from build123d import *

# Parameters (mm, degrees)
SKETCH2_R           = 13.5
BOSS_EXTRUDE1_DEPTH = 8
SKETCH5_R           = 2.3
CUT_EXTRUDE4_DEPTH  = 10
SKETCH8_W           = 10
SKETCH8_H           = 1
CUT_EXTRUDE5_DEPTH  = 1
SKETCH11_R          = 3.5
CUT_EXTRUDE6_DEPTH  = 4.32
SKETCH12_R          = 1.27
CUT_EXTRUDE7_DEPTH  = 32.5


with BuildPart() as part:
    # Sketch2 → Boss-Extrude1 (new body)
    with BuildSketch(Plane.XY):
        Circle(SKETCH2_R)
    extrude(amount=BOSS_EXTRUDE1_DEPTH)

    # Sketch5 → Cut-Extrude4 (cut)
    with BuildSketch(Plane.XY.offset(8)):
        with Locations((0, 8)):
            Circle(SKETCH5_R)
    cut_extrude4 = extrude(amount=-CUT_EXTRUDE4_DEPTH, mode=Mode.SUBTRACT)

    # Mirror1: Cut-Extrude4 across plane
    add(cut_extrude4.mirror(Plane.ZX), mode=Mode.SUBTRACT)

    # Sketch8 → Cut-Extrude5 (cut)
    with BuildSketch(Plane(origin=(0, 0, 0), x_dir=(-1, 0, 0), z_dir=(0, 0, -1))):
        with Locations((-13.5, 0)):
            Rectangle(SKETCH8_W, SKETCH8_H)
    cut_extrude5 = extrude(amount=-CUT_EXTRUDE5_DEPTH, mode=Mode.SUBTRACT)

    # Mirror2: Cut-Extrude5 across plane
    add(cut_extrude5.mirror(Plane(origin=(0, 0, 0), x_dir=(0, 0, 1), z_dir=(1, 0, 0))), mode=Mode.SUBTRACT)

    # Sketch11 → Cut-Extrude6 (cut)
    with BuildSketch(Plane.XY.offset(8)):
        with Locations((0, 8)):
            Circle(SKETCH11_R)
    cut_extrude6 = extrude(amount=-CUT_EXTRUDE6_DEPTH, mode=Mode.SUBTRACT)

    # Mirror3: Cut-Extrude6 across plane
    add(cut_extrude6.mirror(Plane.ZX), mode=Mode.SUBTRACT)

    # Sketch12 → Cut-Extrude7 (cut)
    with BuildSketch(Plane.XY.offset(8)):
        with Locations((4.89, 0)):
            Circle(SKETCH12_R)
        with Locations((-4.89, 0)):
            Circle(SKETCH12_R)
    extrude(amount=-CUT_EXTRUDE7_DEPTH, mode=Mode.SUBTRACT)


solid = part.part
Design review of the part built by this model. Coordinates are the model's own, in mm. A direction names the side the tool comes from. Give positions to 0.01 mm unless a question says otherwise; leave off trailing zeros. Loops run counter-clockwise (first coordinate to the right, second up) from the corner with the lowest first, then second, coordinate; pieces in that order, holes last. Notation, with made-up numbers: M 20,73.5 L 36,73.5 A24 ccw 36,92.5 Z; hole C -32,36.5 d8. An arc over 180 degrees is marked long. Answer as a JSON object with one key per item and string values.
Item 1: Mouldability with a two-part tool opening along Y and no side actions: class faces 5 (the face through (0, 0, 0)), 6 (the face through (11, 0, 1)), 7 (the face through (-2.93, -13.18, 3.94)) as pulls with the +Y half, pulls with the -Y half, needs draft (parallel to the pull), parting line crosses it, or undercut.
Output values:
{"face 5": "needs draft", "face 6": "undercut", "face 7": "parting line crosses it"}
Item 2: Wall thickness on line 1 along Y through (x, z) = (0, 2.5); line 2 along Y through (x, z) = (0, 5.35); line 3 along X through (y, z) = (5.25, 5.75): over which ranges is each line inside the solid? List them lowest first.
Output values:
{"line 1": "y = -13.5 to -10.3, -5.7 to 5.7, 10.3 to 13.5", "line 2": "y = -13.5 to -11.5, -4.5 to 4.5, 11.5 to 13.5", "line 3": "x = -12.44 to -2.17, 2.17 to 12.44"}
Item 3: Machinability: for faces 1 (the face through (8.5, 0, 0.5)), 2 (the face through (-11, 0, 1)), 3 (the face through (-0.759, 4.583, 5.87)), 4 (the face through (-3.68, 0.38, 4.06)), which of the approach directions +Z, -Z, +X, -X, +Y, -Y give a long, thin tool a straight path to every point of the face, cutting with its end or side? Answer none if there is none.
Output values:
{"face 1": "-Z, +X", "face 2": "-Z, -X", "face 3": "+Z", "face 4": "+Z, -Z"}
Item 4: We need section D-D (x = -5.75). State the section outline as (y, z) points.
Output values:
{"outline": "M -12.21,0 L -0.93,0 L -0.93,8 L -12.21,8 Z; M 0.93,0 L 12.21,0 L 12.21,8 L 0.93,8 Z"}
Item 5: We need section A-A (x = 0). State the section outline as (y, z) points, and give its area (3 significant figures).
Output values:
{"outline": "M -13.5,0 L -10.3,0 L -10.3,3.68 L -11.5,3.68 L -11.5,8 L -13.5,8 Z; M -5.7,0 L 5.7,0 L 5.7,3.68 L 4.5,3.68 L 4.5,8 L -4.5,8 L -4.5,3.68 L -5.7,3.68 Z; M 10.3,0 L 13.5,0 L 13.5,8 L 11.5,8 L 11.5,3.68 L 10.3,3.68 Z", "area": "122 mm2"}
Item 6: We need section B-B (y = 0). State the section outline as (x, z) points.
Output values:
{"outline": "M -13.5,1 L -8.5,1 L -8.5,0 L -6.16,0 L -6.16,8 L -13.5,8 Z; M -3.62,0 L 3.62,0 L 3.62,8 L -3.62,8 Z; M 6.16,0 L 8.5,0 L 8.5,1 L 13.5,1 L 13.5,8 L 6.16,8 Z"}
Item 7: We need section C-C (z = 6.75). State the section outline as (x, y) points.
Output values:
{"outline": "C 0,0 d27; hole C -4.89,0 d2.54; hole C 0,-8 d7; hole C 0,8 d7; hole C 4.89,0 d2.54"}
Item 8: For P1, Ø0.8, axis at y = 0, z = 0.5, coming from the +X side; P2, Ø2, axis at x = 0.5, y = 6.5, coming from the +Z side; P3, Ø0.5, axis at y = 0, z = 0.5, coming from the -X side, all flat-tipped, find the tip position at first contact; note any pin that passes through.
Output values:
{"P1": "stops at x = 8.5", "P2": "stops at z = 3.68", "P3": "stops at x = -8.5"}
